Here's how the part is built. I have some questions about the finished solid (model axes, mm). Round coordinates to 2 decimals unless told otherwise and drop trailing zeros. Write each loop counter-clockwise with the first axis right and the second up, starting at its lowest first coordinate (ties: lowest second). Pieces come first, ordered by that corner, then holes. Notation, with made-up numbers: (54, 41) -> (58, 41) arc R24 ccw to (58, 56) -> close; hole circle Ø3 at (77.5, 11.5). An arc over 180 degrees is marked (long way). Answer in a Markdown table with one row per item. Add a question column.
from build123d import *

# Parameters (mm, degrees)
F0_R     = 1.85
F0_R_2   = 6.375
F0_R_3   = 1.3716
F1_DEPTH = 3.2004


with BuildPart() as f1:
    # F0 (on Front) → F1 (new body)
    with BuildSketch(Plane.XZ):
        with BuildLine():
            ThreePointArc((-79.689629, -272.1204697257), (-78.9456802243, -273.91652095), (-77.149629, -274.6604697257))
            Line((-77.149629, -274.6604697257), (-3.589629, -274.6604697257))
            ThreePointArc((-3.589629, -274.6604697257), (-1.7935777758, -273.9165209499), (-1.049629, -272.1204697257))
            Line((-1.049629, -272.1204697257), (-1.049629, -99.4004697257))
            ThreePointArc((-1.049629, -99.4004697257), (-1.7935777758, -97.6044185016), (-3.589629, -96.8604697257))
            Line((-3.589629, -96.8604697257), (-20.354629, -96.8604697257))
            Line((-20.354629, -96.8604697257), (-20.354629, -78.0314697257))
            ThreePointArc((-20.354629, -78.0314697257), (-21.0985777758, -76.2354185016), (-22.894629, -75.4914697257))
            Line((-22.894629, -75.4914697257), (-57.844629, -75.4914697257))
            ThreePointArc((-57.844629, -75.4914697257), (-59.6406802243, -76.2354185015), (-60.384629, -78.0314697257))
            Line((-60.384629, -78.0314697257), (-60.384629, -96.8604697257))
            Line((-60.384629, -96.8604697257), (-77.149629, -96.8604697257))
            ThreePointArc((-77.149629, -96.8604697257), (-78.9456802243, -97.6044185015), (-79.689629, -99.4004697257))
            Line((-79.689629, -99.4004697257), (-79.689629, -272.1204697257))
        make_face()
        with BuildLine():
            Line((-67.5448753625, -255.545025575), (-67.5448753625, -256.4746303251))
            Line((-67.5448753625, -256.4746303251), (-70.1828327017, -256.808961858))
            Line((-70.1828327017, -256.808961858), (-70.1828327017, -271.2830709061))
            Line((-70.1828327017, -271.2830709061), (-66.7049693163, -271.2830709061))
            add(Edge.make_bspline(
                [(-66.7049693163, -271.2830709061), (-63.9895449146, -271.2830709061), (-62.7133769901, -271.0262064356)],
                knots=[0, 0, 0, 1, 1, 1], degree=2))
            Line((-62.7133769901, -271.0262064356), (-61.6696102531, -267.4708759878))
            Line((-61.6696102531, -267.4708759878), (-60.5239131707, -267.4708759878))
            Line((-60.5239131707, -267.4708759878), (-61.0091016149, -272.6326286793))
            Line((-61.0091016149, -272.6326286793), (-76.3883521301, -272.6326286793))
            Line((-76.3883521301, -272.6326286793), (-76.3883521301, -271.7030239291))
            Line((-76.3883521301, -271.7030239291), (-74.1948110969, -271.3564607548))
            Line((-74.1948110969, -271.3564607548), (-74.1948110969, -256.808961858))
            Line((-74.1948110969, -256.808961858), (-76.3720432749, -256.4746303251))
            Line((-76.3720432749, -256.4746303251), (-76.3720432749, -255.545025575))
            Line((-76.3720432749, -255.545025575), (-67.5448753625, -255.545025575))
        make_face(mode=Mode.SUBTRACT)
        with Locations((-73.079629, -231.3779697257)):
            Circle(F0_R, mode=Mode.SUBTRACT)
        with BuildLine():
            Line((-50.1392495805, -255.545025575), (-50.1392495805, -256.4746303251))
            Line((-50.1392495805, -256.4746303251), (-52.7772069197, -256.808961858))
            Line((-52.7772069197, -256.808961858), (-52.7772069197, -271.2830709061))
            Line((-52.7772069197, -271.2830709061), (-49.2993435343, -271.2830709061))
            add(Edge.make_bspline(
                [(-49.2993435343, -271.2830709061), (-46.5839191327, -271.2830709061), (-45.3077512081, -271.0262064356)],
                knots=[0, 0, 0, 1, 1, 1], degree=2))
            Line((-45.3077512081, -271.0262064356), (-44.2639844712, -267.4708759878))
            Line((-44.2639844712, -267.4708759878), (-43.1182873888, -267.4708759878))
            Line((-43.1182873888, -267.4708759878), (-43.6034758329, -272.6326286793))
            Line((-43.6034758329, -272.6326286793), (-58.9827263482, -272.6326286793))
            Line((-58.9827263482, -272.6326286793), (-58.9827263482, -271.7030239291))
            Line((-58.9827263482, -271.7030239291), (-56.789185315, -271.3564607548))
            Line((-56.789185315, -271.3564607548), (-56.789185315, -256.808961858))
            Line((-56.789185315, -256.808961858), (-58.9664174929, -256.4746303251))
            Line((-58.9664174929, -256.4746303251), (-58.9664174929, -255.545025575))
            Line((-58.9664174929, -255.545025575), (-50.1392495805, -255.545025575))
        make_face(mode=Mode.SUBTRACT)
        with BuildLine():
            add(Edge.make_bspline(
                [(-34.3828567872, -269.9824396987), (-33.345205871, -271.0792102152), (-31.3432938872, -271.0792102152)],
                knots=[0, 0, 0, 1, 1, 1], degree=2))
            add(Edge.make_bspline(
                [(-31.3432938872, -271.0792102152), (-29.4310806073, -271.0792102152), (-28.3873138703, -270.0089415885)],
                knots=[0, 0, 0, 1, 1, 1], degree=2))
            add(Edge.make_bspline(
                [(-28.3873138703, -270.0089415885), (-27.3435471333, -268.9386729617), (-27.3435471333, -266.8592939153)],
                knots=[0, 0, 0, 1, 1, 1], degree=2))
            Line((-27.3435471333, -266.8592939153), (-27.3435471333, -256.808961858))
            Line((-27.3435471333, -256.808961858), (-29.6349412981, -256.4746303251))
            Line((-29.6349412981, -256.4746303251), (-29.6349412981, -255.545025575))
            Line((-29.6349412981, -255.545025575), (-23.8249116098, -255.545025575))
            Line((-23.8249116098, -255.545025575), (-23.8249116098, -256.4746303251))
            Line((-23.8249116098, -256.4746303251), (-25.7615881726, -256.808961858))
            Line((-25.7615881726, -256.808961858), (-25.7615881726, -266.7573635699))
            add(Edge.make_bspline(
                [(-25.7615881726, -266.7573635699), (-25.7615881726, -269.7133435868), (-27.4699407616, -271.2932639406)],
                knots=[0, 0, 0, 1, 1, 1], degree=2))
            add(Edge.make_bspline(
                [(-27.4699407616, -271.2932639406), (-29.1782933507, -272.8731842944), (-32.3503656998, -272.8731842944)],
                knots=[0, 0, 0, 1, 1, 1], degree=2))
            add(Edge.make_bspline(
                [(-32.3503656998, -272.8731842944), (-35.7793025193, -272.8731842944), (-37.607932916, -271.2749164784)],
                knots=[0, 0, 0, 1, 1, 1], degree=2))
            add(Edge.make_bspline(
                [(-37.607932916, -271.2749164784), (-39.4365633126, -269.6766486624), (-39.4365633126, -266.6554332245)],
                knots=[0, 0, 0, 1, 1, 1], degree=2))
            Line((-39.4365633126, -266.6554332245), (-39.4365633126, -256.808961858))
            Line((-39.4365633126, -256.808961858), (-41.3732398754, -256.4746303251))
            Line((-41.3732398754, -256.4746303251), (-41.3732398754, -255.545025575))
            Line((-41.3732398754, -255.545025575), (-33.2310438841, -255.545025575))
            Line((-33.2310438841, -255.545025575), (-33.2310438841, -256.4746303251))
            Line((-33.2310438841, -256.4746303251), (-35.4205077035, -256.808961858))
            Line((-35.4205077035, -256.808961858), (-35.4205077035, -266.8348306324))
            add(Edge.make_bspline(
                [(-35.4205077035, -266.8348306324), (-35.4205077035, -268.8856691821), (-34.3828567872, -269.9824396987)],
                knots=[0, 0, 0, 1, 1, 1], degree=2))
        make_face(mode=Mode.SUBTRACT)
        with Locations((-40.364429, -231.3788697257)):
            Circle(F0_R_2, mode=Mode.SUBTRACT)
        Polygon((-9.656593598, -255.545025575), (-4.6253117486, -255.545025575), (-4.6253117486, -256.4746303251), (-6.2439656337, -256.8211934995), (-12.8449748024, -273.0281184195), (-14.5370185362, -273.0281184195), (-21.4805136654, -256.8211934995), (-22.8830752182, -256.4746303251), (-22.8830752182, -255.545025575), (-15.4543916449, -255.545025575), (-15.4543916449, -256.4746303251), (-17.227979655, -256.8211934995), (-12.4209445655, -268.021299853), (-7.9360093675, -256.8211934995), (-9.656593598, -256.4746303251), align=None, mode=Mode.SUBTRACT)
        with Locations((-7.659629, -231.3779697257)):
            Circle(F0_R, mode=Mode.SUBTRACT)
        with Locations((-76.184429, -149.3622697257)):
            Circle(F0_R_3, mode=Mode.SUBTRACT)
        with Locations((-76.184429, -100.3656697257)):
            Circle(F0_R_3, mode=Mode.SUBTRACT)
        with Locations((-55.482429, -92.6280697257)):
            Circle(F0_R, mode=Mode.SUBTRACT)
        with Locations((-55.482429, -80.4614697257)):
            Circle(F0_R, mode=Mode.SUBTRACT)
        with Locations((-18.196229, -149.3622697257)):
            Circle(F0_R_3, mode=Mode.SUBTRACT)
        with Locations((-25.256829, -92.6280697257)):
            Circle(F0_R, mode=Mode.SUBTRACT)
        with Locations((-25.256829, -80.4614697257)):
            Circle(F0_R, mode=Mode.SUBTRACT)
        with Locations((-18.196229, -100.3656697257)):
            Circle(F0_R_3, mode=Mode.SUBTRACT)
    extrude(amount=F1_DEPTH)


solid = f1.part
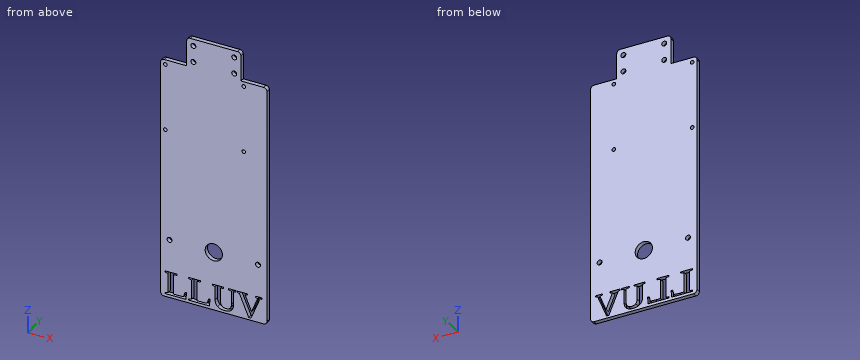
Item 1: For P1, Ø4, axis at x = -38, z = -246, coming from the +Y side, with a flat end and sliding along its axis, tell me the tip position at first contact or that it passes through.
Item 2: If we section it at A-A on z = -88.5: Please give me the cut outline in (x, y).
Item 3: I need wall thicknesses on line 1 along Z through (x, y) = (-56.5, -2.65); line 2 along Z through (x, y) = (-75.5, -2.8); line 3 along Z through (x, y) = (-63, -0.5). Which ranges of each line are inside material? Lowest first, please. Write a range as from..to.
Item 4: If we section it at B-B on y = -2.4: Give the number of separate pieces and of enclosed holes in the cut face, then the cut area to 3 significant figures.
Results list:
| question | item | result |
|---|---|---|
| 1 | P1 | y = 0 |
| 2 | outline | (-60.38, -3.2) -> (-20.35, -3.2) -> (-20.35, 0) -> (-60.38, 0) -> close |
| 3 | line 1 | -274.66..-272.63, -255.55..-94.17, -91.08..-82.01, -78.92..-75.49 |
| 3 | line 2 | -274.66..-272.63, -271.56..-256.61, -255.55..-150.55, -148.17..-101.55, -99.18..-96.86 |
| 3 | line 3 | -274.66..-272.63, -271.08..-96.86 |
| 4 | separate pieces | 1 |
| 4 | enclosed holes | 15 |
| 4 | area | 14,200 mm² |
